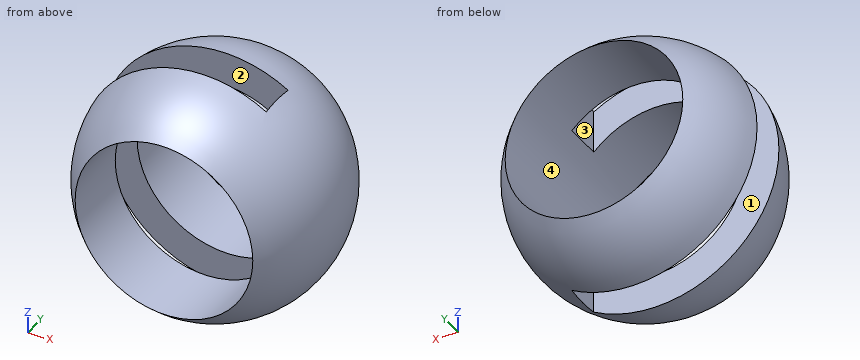
from build123d import *

# Parameters (mm, degrees)
CROQUIS3_W                 = 20
CROQUIS3_H                 = 6
CROQUIS4_W                 = 20
CROQUIS4_H                 = 6
CROQUIS8_R                 = 14.282856857
CORTAR_EXTRUIR2_DEPTH      = 40.799497484
CORTAR_EXTRUIR3_DEPTH      = 34
CORTAR_EXTRUIR3_DEPTH_BACK = 34
ESCALA1_SCALE              = 5


with BuildPart() as part:
    # Croquis1 → Revoluci_n1 (revolve)
    with BuildSketch(Plane.XY):
        with BuildLine():
            Line((0, 20), (0, -20))
            ThreePointArc((0, -20), (20, 0), (0, 20))
        make_face()
    revolve(axis=Axis((0, 27.452088109, 0), (0, -1, 0)))

    # Croquis3 → Cortar-Revoluci_n1 (revolve, cut)
    with BuildSketch(Plane.XY, mode=Mode.PRIVATE) as cortar_revoluci_n1_sk:
        with Locations((-10, 17)):
            Rectangle(CROQUIS3_W, CROQUIS3_H)
    revolve(cortar_revoluci_n1_sk.sketch.rotate(Axis((0, 20, 0), (0, -1, 0)), 180), axis=Axis((0, 20, 0), (0, -1, 0)), mode=Mode.SUBTRACT)

    # Croquis4 → Cortar-Revoluci_n2 (revolve, cut)
    with BuildSketch(Plane.XY):
        with Locations((10, -17)):
            Rectangle(CROQUIS4_W, CROQUIS4_H)
    revolve(axis=Axis((0, 0, 0), (0, -1, 0)), mode=Mode.SUBTRACT)

    # Croquis8 → Cortar-Extruir2 (cut, through all)
    with BuildSketch(Plane(origin=(0, 14, 0), x_dir=(1, 0, 0), z_dir=(0, 1, 0))):
        Circle(CROQUIS8_R)
    extrude(amount=-CORTAR_EXTRUIR2_DEPTH, mode=Mode.SUBTRACT)

    # Croquis9 → Cortar-Extruir3 (cut, two sides: drawn at the far end of the back side and taken through both)
    with BuildSketch(Plane.XY.offset(-CORTAR_EXTRUIR3_DEPTH_BACK)):
        Polygon((-20, -3), (10, -3), (10, 0), (10, 3), (-20, 3), align=None)
    extrude(amount=CORTAR_EXTRUIR3_DEPTH + CORTAR_EXTRUIR3_DEPTH_BACK, mode=Mode.SUBTRACT)


with BuildPart() as part_1:
    # Escala1: scaled about (0, 0, 0)
    add(part.part.scale(ESCALA1_SCALE))


solid = part_1.part
Geometry: final body of the model. Coordinates: model frame, mm. Face numbers are marked on the shaded views. A direction names the side the tool comes from. Round coordinates to 2 decimals unless told otherwise and drop trailing zeros. Order: outer loops, then holes, each group sorted by start corner. A loop starts at its lowest first (then second) coordinate and runs counter-clockwise, first axis right, second up. Notation, with made-up numbers: (69.5, -30.5) -> (110.5, -30.5) arc R19 cw to (110.5, -21.5) -> close; hole circle Ø6 at (52.25, 87.25). An arc over 180 degrees is marked (long way). Put each result on its own line as item: value. Start each with the question number.
Q1. Section A-A on x = 0. Return the cut outline in (y, z).
Q2. Pull-direction query (Y, two-part tool) for the marked faces 1 and 2; classes: +Y half, -Y half, draft (parallel to the pull), parting line (faces both ways), or undercut.
Q3. Reachability of the marked faces 3 and 4 from +Z, -Z, +X, -X, +Y, -Y: full face, straight path, thin tool, end or side. Return the list, or none.
Q4. Section C-C on x = -59. Return the cut outline in (y, z).
Q5. Line query: probe 1 along Y at (x, z) = (-84, -27.5); probe 2 along Z at (x, y) = (0, -32); probe 3 along Z at (x, y) = (-20.5, -51). Output: solid intervals per line, ascending.
Q6. Section D-D on z = -30.5. Return the cut outline in (x, y).
Q7. Section B-B on z = 0. Return the cut outline in (x, y).
Q8. First-contact query: pin 1 (8 mm diameter, centred on y = -46.5, z = 56.5, fed in from -X); pin 2 (24 mm diameter, centred on y = -4.5, z = 69, fed in from -X); pin 3 (4 mm diameter, centred on x = 9.5, z = -75, fed in from +Y). Flat tips, straight axial feed; report the tip coordinate or a pass-through.
Ans:
1. outline: (-70, -71.41) arc R100 ccw to (-15, -98.87) -> (-15, -71.41) -> close; (-70, 71.41) -> (-15, 71.41) -> (-15, 98.87) arc R100 ccw to start; (15, -98.87) arc R100 ccw to (70, -71.41) -> (15, -71.41) -> close; (15, 71.41) -> (70, 71.41) arc R100 ccw to (15, 98.87) -> close
2. face 1: undercut
2. face 2: undercut
3. face 3: +Z, -Z, -X
3. face 4: +Y, -Y
4. outline: (-70, -40.24) arc R80.74 ccw to (-15, -79.33) -> (-15, -40.24) -> close; (-70, 40.24) -> (-15, 40.24) -> (-15, 79.33) arc R80.74 ccw to start; (15, -79.33) arc R80.74 ccw to (70, -40.24) -> (15, -40.24) -> close; (15, 40.24) -> (70, 40.24) arc R80.74 ccw to (15, 79.33) -> close
5. probe 1: y = -46.77 to -15, 15 to 46.77
5. probe 2: z = -94.74 to -71.41, 71.41 to 94.74
5. probe 3: z = -83.54 to -68.41, 68.41 to 83.54
6. outline: (-94.05, -15) arc R95.24 ccw to (-64.57, -70) -> (-64.57, -15) -> close; (-94.05, 15) -> (-64.57, 15) -> (-64.57, 70) arc R95.24 ccw to start; (64.57, -70) arc R95.24 ccw to (64.57, 70) -> close
7. outline: (-98.87, -15) arc R100 ccw to (-71.41, -70) -> (-71.41, -15) -> close; (-98.87, 15) -> (-71.41, 15) -> (-71.41, 70) arc R100 ccw to start; (71.41, -70) arc R100 ccw to (71.41, 70) -> close
8. pin 1: stops at x = -72.21
8. pin 2: stops at x = -76.04
8. pin 3: stops at y = 67.7
